from build123d import *

# Parameters (mm, degrees)
SKETCH1_R           = 2.5
BOSS_EXTRUDE1_DEPTH = 2.5


with BuildPart() as part:
    # Sketch1 → Boss-Extrude1 (new body)
    with BuildSketch(Plane.XY):
        Polygon((-172.5, 80), (-105, 80), (-105, 82.5), (-35, 82.5), (-35, 80), (35, 80), (35, 82.5), (105, 82.5), (105, 80), (172.5, 80), (172.5, 47.5), (175, 47.5), (175, 17.5), (172.5, 17.5), (172.5, -17.5), (175, -17.5), (175, -47.5), (172.5, -47.5), (172.5, -80), (105, -80), (105, -82.5), (35, -82.5), (35, -80), (-35, -80), (-35, -82.5), (-105, -82.5), (-105, -80), (-172.5, -80), (-172.5, -47.5), (-175, -47.5), (-175, -17.5), (-172.5, -17.5), (-172.5, 17.5), (-175, 17.5), (-175, 47.5), (-172.5, 47.5), align=None)
        with Locations((-70, -61)):
            Circle(SKETCH1_R, mode=Mode.SUBTRACT)
        with Locations((70, -61)):
            Circle(SKETCH1_R, mode=Mode.SUBTRACT)
        with Locations((70, 61)):
            Circle(SKETCH1_R, mode=Mode.SUBTRACT)
        with Locations((-70, 61)):
            Circle(SKETCH1_R, mode=Mode.SUBTRACT)
        with Locations((153.5, -32.5)):
            Circle(SKETCH1_R, mode=Mode.SUBTRACT)
        with Locations((153.5, 32.5)):
            Circle(SKETCH1_R, mode=Mode.SUBTRACT)
        with Locations((-153.5, -32.5)):
            Circle(SKETCH1_R, mode=Mode.SUBTRACT)
        with Locations((-153.5, 32.5)):
            Circle(SKETCH1_R, mode=Mode.SUBTRACT)
    extrude(amount=BOSS_EXTRUDE1_DEPTH)


solid = part.part
For this review, take the finished solid that the model builds, in its own axes (mm). Coordinates: 2 decimals unless noted, no trailing zeros. Loops run counter-clockwise (first coordinate to the right, second up) from the corner with the lowest first, then second, coordinate; pieces in that order, holes last. Notation, with made-up numbers: (-9, 22.25) - (3, 22.25) arc R24 ccw to (3, 50.25) - close; hole circle Ø3 at (73.5, -1.5). An arc over 180 degrees is marked (long way). Return JSON: item names as keys, results as strings.
Item 1: For line 1 (Y direction, x = -153.5, z = 0.95); line 2 (Y direction, x = 70, z = 0.8); line 3 (X direction, y = -33.5, z = 1.5), list the stretches that pass through material, from the lowest coordinate up.
Determined:
{"line 1": "y = -80 to -35, -30 to 30, 35 to 80", "line 2": "y = -82.5 to -63.5, -58.5 to 58.5, 63.5 to 82.5", "line 3": "x = -175 to -155.79, -151.21 to 151.21, 155.79 to 175"}
Item 2: Insertion check: pin 1 (1.5 mm diameter, centred on y = -8, z = 1.5, fed in from -X); pin 2 (1.2 mm diameter, centred on y = -67, z = 1.5, fed in from +X); pin 3 (0.8 mm diameter, centred on x = 135.5, z = 1, fed in from +Y). Each pin has a flat end and moves straight along its axis. Give the tip position at first contact, or say it passes through.
Determined:
{"pin 1": "stops at x = -172.5", "pin 2": "stops at x = 172.5", "pin 3": "stops at y = 80"}
Item 3: Take a section at B-B (x = -25). Give the boundary of the cut face in (y, z), then the cut area to 3 significant figures.
Determined:
{"outline": "(-80, 0) - (80, 0) - (80, 2.5) - (-80, 2.5) - close", "area": "400 mm2"}
Item 4: Take a section at A-A (z = 0.5). State how many separate pieces and enclosed holes the cut face has, then the cut area to 3 significant figures.
Determined:
{"separate pieces": "1", "enclosed holes": "8", "area": "56,000 mm2"}
